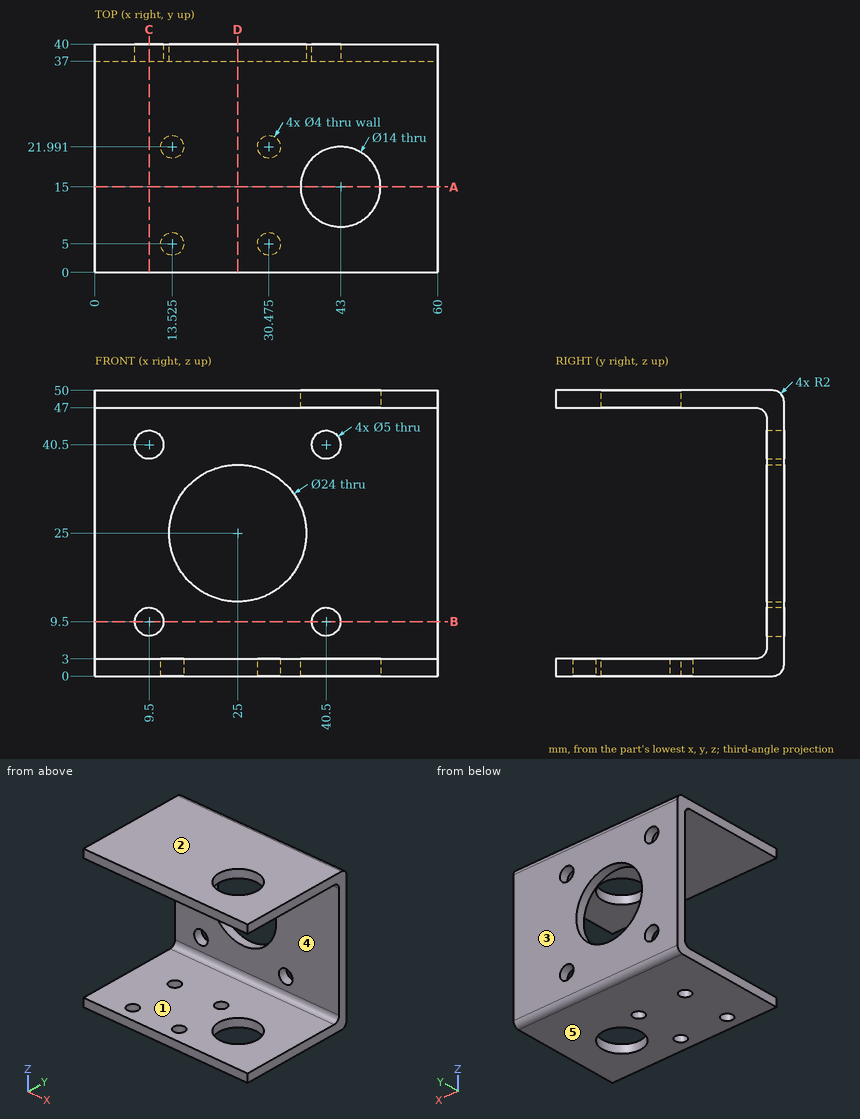
Source: three-view drawing plus pictorial views. Frame: mm from the lowest corner of the part. A direction names the side the tool comes from. Round coordinates to 2 decimals unless told otherwise and drop trailing zeros. Loops run counter-clockwise (first coordinate to the right, second up) from the corner with the lowest first, then second, coordinate; pieces in that order, holes last.
1. Mould query, pull axis Z, two halves, no side actions, for the marked faces 3, 4 and 5. Classes: released by +Z, released by -Z, zero draft, split by the parting line, or undercut.
2. Ray query, L1, parallel to X at y = 39.1, z = 40.5; L2, parallel to Z at x = 55.5, y = 16; L3, parallel to Z at x = 9, y = 39. Return the intervals inside material, ascending.
3. Section query B-B on z = 9.5. Output: boundary loops of the cut face in (x, y).
4. Access query for the marked faces 1 and 2. Directions: +Z, -Z, +X, -X, +Y, -Y. A direction counts if a zero-diameter tool reaches every point of the face in a straight line with its end or side. Return the directions, or none.
5. Section query C-C on x = 9.5. Output: boundary loops of the cut face in (y, z), and give its area (3 significant figures).
6. Section query D-D on x = 25. Output: boundary loops of the cut face in (y, z).
7. Section query A-A on y = 15. Output: boundary loops of the cut face in (x, z), and give its area (3 significant figures).
8. Contact query for flat-ended pins moving along their axis: pin 1 (4 mm diameter, centred on x = 40.5, z = 40.5, fed in from +Y); pin 2 (5 mm diameter, centred on x = 8.5, z = 44, fed in from -Y). Output: stop coordinate, or through.
Answers below:
1. face 3: zero draft
1. face 4: undercut
1. face 5: released by -Z
2. L1: x = 0 to 7, 12 to 38, 43 to 60
2. L2: z = 0 to 3, 47 to 50
2. L3: z = 0.27 to 7.05, 11.95 to 38.05, 42.95 to 49.73
3. outline: (0, 37) - (7, 37) - (7, 40) - (0, 40) - close; (12, 37) - (38, 37) - (38, 40) - (12, 40) - close; (43, 37) - (60, 37) - (60, 40) - (43, 40) - close
4. face 1: +X, -X, -Y
4. face 2: +Z, +X, -X, +Y, -Y
5. outline: (0, 0) - (38, 0) arc R2 ccw to (40, 2) - (40, 7) - (37, 7) - (37, 5) arc R2 cw to (35, 3) - (0, 3) - close; (0, 47) - (35, 47) arc R2 cw to (37, 45) - (37, 43) - (40, 43) - (40, 48) arc R2 ccw to (38, 50) - (0, 50) - close; (37, 12) - (40, 12) - (40, 38) - (37, 38) - close
5. area: 342 mm2
6. outline: (0, 0) - (38, 0) arc R2 ccw to (40, 2) - (40, 13) - (37, 13) - (37, 5) arc R2 cw to (35, 3) - (0, 3) - close; (0, 47) - (35, 47) arc R2 cw to (37, 45) - (37, 37) - (40, 37) - (40, 48) arc R2 ccw to (38, 50) - (0, 50) - close
7. outline: (0, 0) - (36, 0) - (36, 3) - (0, 3) - close; (0, 47) - (36, 47) - (36, 50) - (0, 50) - close; (50, 0) - (60, 0) - (60, 3) - (50, 3) - close; (50, 47) - (60, 47) - (60, 50) - (50, 50) - close
7. area: 276 mm2
8. pin 1: passes through
8. pin 2: stops at y = 36.32
